```python
from build123d import *

# Parameters (mm, degrees)
SKETCH1_R           = 7.15
BOSS_EXTRUDE1_DEPTH = 49
SKETCH2_R           = 2.75
BOSS_EXTRUDE2_DEPTH = 1
FILLET1_R           = 0.3
SKETCH3_R           = 5
BOSS_EXTRUDE3_DEPTH = 1
FILLET3_R           = 0.1


with BuildPart() as part:
    # Sketch1 → Boss-Extrude1 (new body)
    with BuildSketch(Plane(origin=(0, 0, 0), x_dir=(1, 0, 0), z_dir=(0, 1, 0))):
        Circle(SKETCH1_R)
    extrude(amount=BOSS_EXTRUDE1_DEPTH)

    # Sketch2 → Boss-Extrude2 (add)
    with BuildSketch(Plane(origin=(0, 49, 0), x_dir=(1, 0, 0), z_dir=(0, 1, 0))):
        Circle(SKETCH2_R)
    extrude(amount=BOSS_EXTRUDE2_DEPTH)

    # Fillet1
    fillet1_edges = [part.edges().sort_by_distance(p)[0] for p in [
        (-7.15, 0, 0),
        (-7.15, 49, 0),
        (-2.75, 50, 0),
    ]]
    fillet(fillet1_edges, radius=FILLET1_R)

    # Sketch3 → Boss-Extrude3 (add)
    with BuildSketch(Plane.XZ):
        Circle(SKETCH3_R)
    extrude(amount=BOSS_EXTRUDE3_DEPTH)

    # Fillet3
    fillet3_edges = [part.edges().sort_by_distance(p)[0] for p in [
        (-5, -1, 0),
    ]]
    fillet(fillet3_edges, radius=FILLET3_R)


solid = part.part
```
Can you work these out from the model? Positions are in its coordinate system, mm. A direction names the side the tool comes from. Give positions to 0.01 mm unless a question says otherwise; leave off trailing zeros. Order: outer loops, then holes, each group sorted by start corner. A loop starts at its lowest first (then second) coordinate and runs counter-clockwise, first axis right, second up. Notation, with made-up numbers: (86.25, 8.25) - (99.25, 8.25) arc R16 cw to (99.25, 31.25) - close; hole circle Ø10 at (40.5, 52.25). An arc over 180 degrees is marked (long way). Use a Markdown table: item, result. Add a question column.
Q1. I'm going to push flat-ended pins straight in: pin 1 (5 mm diameter, centred on x = 3.5, y = 25.5, fed in from -Z); pin 2 (1 mm diameter, centred on x = 3, z = 5, fed in from +Y); pin 3 (3 mm diameter, centred on x = -4, y = 17.5, fed in from -Z). Where does each tip first touch, or does it pass through?
Q2. Please list where these lines run through material, in increasing order: line 1 along Y through (x, z) = (5, -1); line 2 along Y through (x, z) = (2.75, 0.75); line 3 along X through (y, z) = (12.5, 0.25).
Q3. If we section it at C-C on y = 18.5: Write out the boundary of the cut face in (x, z).
Q4. If we section it at A-A on z = 0: Write out the boundary of the cut face in (x, y).
Q5. If we section it at B-B on x = 0: Write out the boundary of the cut face in (y, z).
Q6. On a 3-axis mill with a long thin cutter (end or side, diameter ignored), from which of +Z, -Z, +X, -X, +Y, -Y can I reach the whole of each face in a straight line? I mean faces 1 (the flat face through (3, 49, 0)), 2 (the flat face through (0, -1, 0)), 3 (the flat face through (-5, 0, 2)). Say none if no direction works.
Answers follow:
| question | item | result |
|---|---|---|
| 1 | pin 1 | stops at z = -7.08 |
| 1 | pin 2 | stops at y = 49 |
| 1 | pin 3 | stops at z = -6.7 |
| 2 | line 1 | y = 0 to 49 |
| 2 | line 2 | y = -1 to 49 |
| 2 | line 3 | x = -7.15 to 7.15 |
| 3 | outline | circle Ø14.3 at (0, 0) |
| 4 | outline | (-7.15, 0.3) arc R0.3 ccw to (-6.85, 0) - (-5, 0) - (-5, -0.9) arc R0.1 ccw to (-4.9, -1) - (4.9, -1) arc R0.1 ccw to (5, -0.9) - (5, 0) - (6.85, 0) arc R0.3 ccw to (7.15, 0.3) - (7.15, 48.7) arc R0.3 ccw to (6.85, 49) - (2.75, 49) - (2.75, 49.7) arc R0.3 ccw to (2.45, 50) - (-2.45, 50) arc R0.3 ccw to (-2.75, 49.7) - (-2.75, 49) - (-6.85, 49) arc R0.3 ccw to (-7.15, 48.7) - close |
| 5 | outline | (-1, -4.9) arc R0.1 ccw to (-0.9, -5) - (0, -5) - (0, -6.85) arc R0.3 ccw to (0.3, -7.15) - (48.7, -7.15) arc R0.3 ccw to (49, -6.85) - (49, -2.75) - (49.7, -2.75) arc R0.3 ccw to (50, -2.45) - (50, 2.45) arc R0.3 ccw to (49.7, 2.75) - (49, 2.75) - (49, 6.85) arc R0.3 ccw to (48.7, 7.15) - (0.3, 7.15) arc R0.3 ccw to (0, 6.85) - (0, 5) - (-0.9, 5) arc R0.1 ccw to (-1, 4.9) - close |
| 6 | face 1 | +Y |
| 6 | face 2 | +Z, -Z, +X, -X, -Y |
| 6 | face 3 | -Y |
